```python
from build123d import *

# Parameters (mm, degrees)
SKETCH1_R           = 27.5
SKETCH1_R_2         = 25
BOSS_EXTRUDE1_DEPTH = 25
SKETCH2_R           = 25
BOSS_EXTRUDE2_DEPTH = 2.5
BOSS_EXTRUDE3_START = 0.5
SKETCH3_R           = 7.25
BOSS_EXTRUDE3_DEPTH = 8
SKETCH3_3_R         = 9.25
SKETCH3_3_R_2       = 7.25
BOSS_EXTRUDE4_DEPTH = 8
SKETCH4_R           = 7.25
CUT_EXTRUDE1_DEPTH  = 3
CUT_EXTRUDE3_DEPTH  = 6
SKETCH6_R           = 0.5
SKETCH6_W           = 6
SKETCH6_H           = 6
CUT_EXTRUDE5_DEPTH  = 6.05
SKETCH7_R           = 1.525
CUT_EXTRUDE6_DEPTH  = 6.05


with BuildPart() as part:
    # Sketch1 → Boss-Extrude1 (new body)
    with BuildSketch(Plane(origin=(0, 0, 0), x_dir=(1, 0, 0), z_dir=(0, 1, 0))):
        with Locations(Location((0, 0, 0), (0, 0, 270))):
            Circle(SKETCH1_R)
        with Locations(Location((0, 0, 0), (0, 0, 270))):
            Circle(SKETCH1_R_2, mode=Mode.SUBTRACT)
    extrude(amount=BOSS_EXTRUDE1_DEPTH)

    # Sketch2 → Boss-Extrude2 (add)
    with BuildSketch(Plane.XZ):
        with Locations(Location((0, 0, 0), (0, 0, 270))):
            Circle(SKETCH2_R)
    extrude(amount=-BOSS_EXTRUDE2_DEPTH)



with BuildPart() as body_2:
    # Sketch3 → Boss-Extrude3 (new body)
    with BuildSketch(Plane(origin=(0, 2.5, 0), x_dir=(1, 0, 0), z_dir=(0, 1, 0)).offset(BOSS_EXTRUDE3_START)):
        with Locations(Location((0, 0, 0), (0, 0, 270))):
            Circle(SKETCH3_R)
    extrude(amount=BOSS_EXTRUDE3_DEPTH)


with BuildPart() as part_1:
    add(part.part)

    add(body_2.part)  # Boss-Extrude4 merges body 2
    # Sketch3_3 → Boss-Extrude4 (add)
    with BuildSketch(Plane(origin=(0, 2.5, 0), x_dir=(1, 0, 0), z_dir=(0, 1, 0))):
        with Locations(Location((0, 0, 0), (0, 0, 90))):
            Circle(SKETCH3_3_R)
        with Locations(Location((0, 0, 0), (0, 0, 270))):
            Circle(SKETCH3_3_R_2, mode=Mode.SUBTRACT)
    extrude(amount=BOSS_EXTRUDE4_DEPTH)

    # Sketch4 → Cut-Extrude1 (cut)
    with BuildSketch(Plane.XZ):
        with Locations(Location((0, 0, 0), (0, 0, 90))):
            Circle(SKETCH4_R)
    extrude(amount=-CUT_EXTRUDE1_DEPTH, mode=Mode.SUBTRACT)

    # Sketch5 → Cut-Extrude3 (cut)
    with BuildSketch(Plane.XZ):
        with BuildLine():
            Line((11.813657351, -3), (20.645822822, -3))
            ThreePointArc((20.645822822, -3), (23.044950571, -4.198837585), (23.526635309, -6.837209302))
            ThreePointArc((23.526635309, -6.837209302), (17.324116139, -17.324116139), (6.837209302, -23.526635309))
            ThreePointArc((6.837209302, -23.526635309), (4.198837585, -23.044950571), (3, -20.645822822))
            Line((3, -20.645822822), (3, -11.813657351))
            ThreePointArc((3, -11.813657351), (3.443100344, -10.244497018), (4.641509434, -9.138867007))
            ThreePointArc((4.641509434, -9.138867007), (7.247844507, -7.247844507), (9.138867007, -4.641509434))
            ThreePointArc((9.138867007, -4.641509434), (10.244497018, -3.443100344), (11.813657351, -3))
        make_face()
        with BuildLine():
            Line((-3, -11.813657351), (-3, -20.645822822))
            ThreePointArc((-3, -20.645822822), (-4.198837585, -23.044950571), (-6.837209302, -23.526635309))
            ThreePointArc((-6.837209302, -23.526635309), (-17.324116139, -17.324116139), (-23.526635309, -6.837209302))
            ThreePointArc((-23.526635309, -6.837209302), (-23.044950571, -4.198837585), (-20.645822822, -3))
            Line((-20.645822822, -3), (-11.813657351, -3))
            ThreePointArc((-11.813657351, -3), (-10.244497018, -3.443100344), (-9.138867007, -4.641509434))
            ThreePointArc((-9.138867007, -4.641509434), (-7.247844507, -7.247844507), (-4.641509434, -9.138867007))
            ThreePointArc((-4.641509434, -9.138867007), (-3.443100344, -10.244497018), (-3, -11.813657351))
        make_face()
        with BuildLine():
            Line((-11.813657351, 3), (-20.645822822, 3))
            ThreePointArc((-20.645822822, 3), (-23.044950571, 4.198837585), (-23.526635309, 6.837209302))
            ThreePointArc((-23.526635309, 6.837209302), (-17.324116139, 17.324116139), (-6.837209302, 23.526635309))
            ThreePointArc((-6.837209302, 23.526635309), (-4.198837585, 23.044950571), (-3, 20.645822822))
            Line((-3, 20.645822822), (-3, 11.813657351))
            ThreePointArc((-3, 11.813657351), (-3.443100344, 10.244497018), (-4.641509434, 9.138867007))
            ThreePointArc((-4.641509434, 9.138867007), (-7.247844507, 7.247844507), (-9.138867007, 4.641509434))
            ThreePointArc((-9.138867007, 4.641509434), (-10.244497018, 3.443100344), (-11.813657351, 3))
        make_face()
        with BuildLine():
            Line((3, 11.813657351), (3, 20.645822822))
            ThreePointArc((3, 20.645822822), (4.198837585, 23.044950571), (6.837209302, 23.526635309))
            ThreePointArc((6.837209302, 23.526635309), (17.324116139, 17.324116139), (23.526635309, 6.837209302))
            ThreePointArc((23.526635309, 6.837209302), (23.044950571, 4.198837585), (20.645822822, 3))
            Line((20.645822822, 3), (11.813657351, 3))
            ThreePointArc((11.813657351, 3), (10.244497018, 3.443100344), (9.138867007, 4.641509434))
            ThreePointArc((9.138867007, 4.641509434), (7.247844507, 7.247844507), (4.641509434, 9.138867007))
            ThreePointArc((4.641509434, 9.138867007), (3.443100344, 10.244497018), (3, 11.813657351))
        make_face()
    extrude(amount=-CUT_EXTRUDE3_DEPTH, mode=Mode.SUBTRACT)

    # Sketch6 → Cut-Extrude5 (cut)
    with BuildSketch(Plane.XZ.offset(-3)):
        with Locations((-3, -3)):
            Circle(SKETCH6_R)
        with Locations((3, 3)):
            Circle(SKETCH6_R)
        Rectangle(SKETCH6_W, SKETCH6_H)
        with BuildLine():
            ThreePointArc((2.5, 3), (2.646446609, 2.646446609), (3, 2.5))
            Line((3, 2.5), (3, 3))
            Line((3, 3), (2.5, 3))
        make_face()
        with BuildLine():
            Line((3, 3), (3, 2.5))
            ThreePointArc((3, 2.5), (3.353553391, 2.646446609), (3.5, 3))
            ThreePointArc((3.5, 3), (3, 3.5), (2.5, 3))
            Line((2.5, 3), (3, 3))
        make_face()
        with BuildLine():
            Line((-3, -2.5), (-3, -3))
            Line((-3, -3), (-2.5, -3))
            ThreePointArc((-2.5, -3), (-2.646446609, -2.646446609), (-3, -2.5))
        make_face()
        with BuildLine():
            Line((-2.5, -3), (-3, -3))
            Line((-3, -3), (-3, -2.5))
            ThreePointArc((-3, -2.5), (-3.353553391, -3.353553391), (-2.5, -3))
        make_face()
    extrude(amount=-CUT_EXTRUDE5_DEPTH, mode=Mode.SUBTRACT)

    # Sketch7 → Cut-Extrude6 (cut)
    with BuildSketch(Plane.XZ.offset(-9.05)):
        with Locations(Location((0, 0, 0), (0, 0, 270))):
            Circle(SKETCH7_R)
    extrude(amount=-CUT_EXTRUDE6_DEPTH, mode=Mode.SUBTRACT)


solid = part_1.part
```
CAD build for the part. Positions are in the model's coordinates, mm. A direction names the side the tool comes from. Coordinates: 2 decimals unless noted, no trailing zeros. Order: outer loops, then holes, each group sorted by start corner. A loop starts at its lowest first (then second) coordinate and runs counter-clockwise, first axis right, second up.
(1) Saw through at D-D, the plane z = 10. Write the cut outline in (x, y), and give its area (3 significant figures).
Solution:
outline: (-25.62, 0) - (-22.37, 0) - (-22.37, 2.5) - (-22.91, 2.5) - (-22.91, 25) - (-25.62, 25) - close; (-3.61, 0) - (3.61, 0) - (3.61, 2.5) - (-3.61, 2.5) - close; (22.37, 0) - (25.62, 0) - (25.62, 25) - (22.91, 25) - (22.91, 2.5) - (22.37, 2.5) - close
area: 156 mm2
(2) Saw through at A-A, the plane y = 8. Write the cut outline in (x, z).
Solution:
outline: circle Ø55 at (0, 0); circle Ø18.5 at (0, 0); hole circle Ø50 at (0, 0); hole (-3, -2.5) arc R0.5 ccw (long way) to (-2.5, -3) - (3, -3) - (3, 2.5) arc R0.5 ccw (long way) to (2.5, 3) - (-3, 3) - close
(3) Saw through at C-C, the plane x = 16.5. Write the cut outline in (y, z), and give its area (3 significant figures).
Solution:
outline: (0, -22) - (25, -22) - (25, -18.78) - (2.5, -18.78) - (2.5, -18.11) - (0, -18.11) - close; (0, -3) - (2.5, -3) - (2.5, 3) - (0, 3) - close; (0, 18.11) - (2.5, 18.11) - (2.5, 18.78) - (25, 18.78) - (25, 22) - (0, 22) - close
area: 179 mm2
(4) Saw through at B-B, the plane z = 0. Write the cut outline in (x, y) (3 decimals).
Solution:
outline: (-27.5, 0) - (-7.25, 0) - (-7.25, 3) - (-3, 3) - (-3, 9.05) - (-1.525, 9.05) - (-1.525, 11) - (-7.25, 11) - (-7.25, 10.5) - (-9.25, 10.5) - (-9.25, 2.5) - (-25, 2.5) - (-25, 25) - (-27.5, 25) - close; (1.525, 9.05) - (3, 9.05) - (3, 3) - (7.25, 3) - (7.25, 0) - (27.5, 0) - (27.5, 25) - (25, 25) - (25, 2.5) - (9.25, 2.5) - (9.25, 10.5) - (7.25, 10.5) - (7.25, 11) - (1.525, 11) - close
(5) Pin check, flat tips, straight feed: pin 1 Ø1.6 at (y, z) = (5.5, 0.5) entering from +X; pin 2 Ø1.6 at (x, y) = (-1.5, 6) entering from -Z; pin 3 Ø1.2 at (x, y) = (16, 1) entering from +Z; pin 4 Ø16 at (x, z) = (1, -1) entering from -Y. Stop position of each tip, or through.
Solution:
pin 1: stops at x = 27.5
pin 2: stops at z = -27.49
pin 3: stops at z = 22.78
pin 4: stops at y = 0
(6) Drill centre lines: L1, parallel to X at y = 10.65, z = 0 (3 decimals); L2, parallel to Z at x = 0.5, y = 5.5 (3 decimals); L3, parallel to X at y = 16, z = 0. Where is each one in solid material? Low to high.
Solution:
L1: x = -27.5 to -25, -7.25 to -1.525, 1.525 to 7.25, 25 to 27.5
L2: z = -27.495 to -24.995, -9.236 to -3, 3 to 9.236, 24.995 to 27.495
L3: x = -27.5 to -25, 25 to 27.5
(7) Which spindle directions (+Z, -Z, +X, -X, +Y, -Y) get a long thin tool onto all of the face, cutting with end or side? Do faces 1 (the face through (-22.3, 25, 12.1)), 2 (the face through (0.1, 3, -3.3)), 3 (the face through (5, 10.5, 6)), 4 (the face through (10.264, 1.232, 3.431)), 5 (the face through (-6, 0, -6)). Say none if no direction does.
Solution:
face 1: +Z, -Z, +X, -X, +Y
face 2: -Y
face 3: +Y
face 4: +Y, -Y
face 5: +Z, -Z, +X, -X, -Y
